Can you work these out from the model? Positions are in its coordinate system, mm. Face numbers are marked on the shaded views. A direction names the side the tool comes from. Coordinates: 2 decimals unless noted, no trailing zeros. Order: outer loops, then holes, each group sorted by start corner. A loop starts at its lowest first (then second) coordinate and runs counter-clockwise, first axis right, second up.
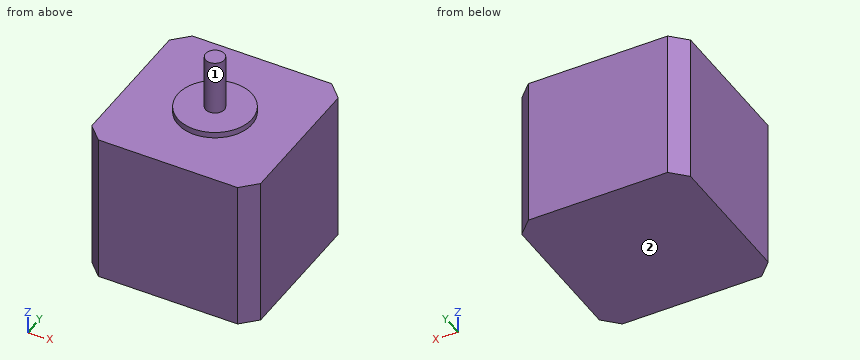
Autodesk Fusion 360 part; units mm, degrees
sketch "Sketch1" plane through (0, 0, 0) normal (0, 0, 1) x (1, 0, 0)
  line L0 (28.5, -28.5) -> (-28.5, -28.5)
  line L1 (-28.5, -28.5) -> (-28.5, 28.5)
  line L2 (-28.5, 28.5) -> (28.5, 28.5)
  line L3 (28.5, 28.5) -> (28.5, -28.5)
  line L4 (28.5, -28.5) -> (-28.5, 28.5) construction
  line L5 (-28.5, -28.5) -> (28.5, 28.5) construction
  dimension "d1" = 57
  dimension "d2" = 57
extrude "Extrude1" add sketch "Sketch1" along normal blind 51
chamfer "Chamfer1" distance 5 angle 45 4 edges at (-28.5, -28.5, 25.5) (28.5, -28.5, 25.5) (-28.5, 28.5, 25.5) (28.5, 28.5, 25.5)
sketch "Sketch2" plane through (0, 0, 51) normal (0, 0, 1) x (-1, 0, 0)
  line L0 (-28.5, -23.5) -> (-23.5, -28.5)
  line L1 (-23.5, -28.5) -> (23.5, -28.5)
  line L2 (23.5, -28.5) -> (28.5, -23.5)
  line L3 (28.5, -23.5) -> (28.5, 23.5)
  line L4 (28.5, 23.5) -> (23.5, 28.5)
  line L5 (23.5, 28.5) -> (-23.5, 28.5)
  line L6 (-23.5, 28.5) -> (-28.5, 23.5)
  line L7 (-28.5, 23.5) -> (-28.5, -23.5)
  circle A0 centre (0, 0) radius 12.5
  circle A1 centre (0, 0) radius 3.175
  dimension "d6" = 25
  dimension "d7" = 6.35
extrude "Extrude2" add sketch "Sketch2" along normal blind 2 contours A0
extrude "Extrude3" add 1 faces at (1.0904, 0.6963, 51) along direction (0, 0, 1) blind 20.6
1. Please list where these lines run through material, in increasing order: probe 1 along Z at (x, y) = (-20, 15.5); probe 2 along Z at (x, y) = (-1, -9.5); probe 3 along Y at (x, z) = (2, 56.5).
Completed:
probe 1: z = 0 to 51
probe 2: z = 0 to 53
probe 3: y = -2.47 to 2.47
2. Imagine slicing it at B-B on z = 16.5. Please give me the cut outline in (x, y), then the cut area to 3 significant figures.
Completed:
outline: (-28.5, -23.5) - (-23.5, -28.5) - (23.5, -28.5) - (28.5, -23.5) - (28.5, 23.5) - (23.5, 28.5) - (-23.5, 28.5) - (-28.5, 23.5) - close
area: 3,200 mm2
3. Imagine slicing it at A-A on y = 0. Please give me the cut outline in (x, z) (3 decimals).
Completed:
outline: (-28.5, 0) - (28.5, 0) - (28.5, 51) - (12.5, 51) - (12.5, 53) - (3.175, 53) - (3.175, 71.6) - (-3.175, 71.6) - (-3.175, 53) - (-12.5, 53) - (-12.5, 51) - (-28.5, 51) - close
4. I'm going to push a flat-ended pin straight in: pin 1 (1 mm diameter, centred on x = -5.5, y = -22, fed in from +Z). Where does the tip first touch, or does it pass through?
Completed:
pin 1: stops at z = 51
5. Imagine slicing it at D-D on y = 8.5. Please give me the cut outline in (x, z), then the cut area to 3 significant figures.
Completed:
outline: (-28.5, 0) - (28.5, 0) - (28.5, 51) - (9.17, 51) - (9.17, 53) - (-9.17, 53) - (-9.17, 51) - (-28.5, 51) - close
area: 2,940 mm2
6. On a 3-axis mill with a long thin cutter (end or side, diameter ignored), from which of +Z, -Z, +X, -X, +Y, -Y can I reach the whole of each face in a straight line? I mean the marked faces 1 and 2. Say none if no direction works.
Completed:
face 1: +Z
face 2: -Z, +X, -X, +Y, -Y
